from build123d import *

# Parameters (mm, degrees)
SKETCH1_R           = 3.2639
BOSS_EXTRUDE1_DEPTH = 0.79375


with BuildPart() as part:
    # Sketch1 → Boss-Extrude1 (new, symmetric)
    with BuildSketch(Plane(origin=(0, 0, 0), x_dir=(0, 0, -1), z_dir=(1, 0, 0))):
        with BuildLine():
            Line((-20.171387669, 38.718044278), (-82.324589357, -6.4389))
            Line((-82.324589357, -6.4389), (-47.512294679, -6.4389))
            Line((-47.512294679, -6.4389), (-47.512294679, -7.23265))
            Line((-47.512294679, -7.23265), (-34.812294679, -7.23265))
            Line((-34.812294679, -7.23265), (-34.812294679, -6.4389))
            Line((-34.812294679, -6.4389), (0, -6.4389))
            ThreePointArc((0, -6.4389), (5.737101909, -2.923199429), (5.209179525, 3.784690461))
            Line((5.209179525, 3.784690461), (-20.171387669, 38.718044278))
        make_face()
        Circle(SKETCH1_R, mode=Mode.SUBTRACT)
    extrude(amount=BOSS_EXTRUDE1_DEPTH, both=True)


solid = part.part
Input: part model. Units: mm. Frame: model coordinates. A direction names the side the tool comes from. Coordinates: 2 decimals unless noted, no trailing zeros. Write each loop counter-clockwise with the first axis right and the second up, starting at its lowest first coordinate (ties: lowest second). Pieces come first, ordered by that corner, then holes. Notation, with made-up numbers: M 52,81 L 103,81 A9 cw 103,94 Z; hole C 67.5,-20 d5. An arc over 180 degrees is marked long. Answer as a JSON object with one key per item and string values. Group by question number.
(1) Section C-C on z = -1. Output: boundary loops of the cut face in (x, y), plus the area to 3 significant figures.
(2) Section D-D on y = 25.5. Output: boundary loops of the cut face in (x, z), plus the area to 3 significant figures.
(3) Set-up query: faces 5 (the face through (0, -6.439, 18)), 6 (the face through (0, -6.439, 65)), 7 (the face through (0.794, 11, 29)). Return all of +Z, -Z, +X, -X, +Y, -Y with unobstructed straight access to the full face (end or side cutting, diameter ignored); none if empty.
(4) Section B-B on y = 0. Output: boundary loops of the cut face in (x, z).
(5) Contact query for flat-ended pins moving along their axis: P1, Ø0.9, axis at x = 0.5, y = -7, coming from the +Z side; P2, Ø0.8, axis at x = 0, z = 16, coming from the -Y side. Output: stop coordinate, or through.
(6) Mould query, pull axis Z, two halves, no side actions, for faces 1 (the face through (0.01, 16.46, 50.81)), 2 (the face through (0.01, -3.01, -5.69)), 3 (the face through (-0.794, 11, 29)), 4 (the face through (-0.011, -3.186, 0.708)). Classes: pulls with the +Z half, pulls with the -Z half, needs draft (parallel to the pull), parting line crosses it, or undercut.
(7) Ray query, line 1 along Y through (x, z) = (0.25, 0); line 2 along Y through (x, z) = (-0.05, 2); line 3 along Z through (x, y) = (-0.2, 3). Return the intervals inside material, ascending. Write a range as [from, to].
(8) Section A-A on x = 0.5. Output: boundary loops of the cut face in (y, z), plus the area to 3 significant figures.
Result set:
{
 "1": {"outline": "M -0.79,-6.36 L 0.79,-6.36 L 0.79,-3.11 L -0.79,-3.11 Z; M -0.79,3.11 L 0.79,3.11 L 0.79,9.58 L -0.79,9.58 Z", "area": "15.4 mm2"},
 "2": {"outline": "M -0.79,10.57 L 0.79,10.57 L 0.79,38.36 L -0.79,38.36 Z", "area": "44.1 mm2"},
 "3": {"face 5": "-Z, +X, -X, -Y", "face 6": "+Z, +X, -X, -Y", "face 7": "+Z, -Z, +X, +Y, -Y"},
 "4": {"outline": "M -0.79,-6.44 L 0.79,-6.44 L 0.79,-3.26 L -0.79,-3.26 Z; M -0.79,3.26 L 0.79,3.26 L 0.79,73.46 L -0.79,73.46 Z"},
 "5": {"P1": "stops at z = 47.51", "P2": "stops at y = -6.44"},
 "6": {"face 1": "pulls with the +Z half", "face 2": "pulls with the -Z half", "face 3": "needs draft", "face 4": "undercut"},
 "7": {"line 1": "y = [-6.44, -3.26], [3.26, 10.95]", "line 2": "y = [-6.44, -2.58], [2.58, 13.71]", "line 3": "z = [-5.7, -1.29], [1.29, 69.33]"},
 "8": {"outline": "M -7.23,34.81 L -6.44,34.81 L -6.44,0 A6.44 ccw 3.78,-5.21 L 38.72,20.17 L -6.44,82.32 L -6.44,47.51 L -7.23,47.51 Z; hole C 0,0 d6.53", "area": "2,080 mm2"}
}
